Read the model definition and answer for the solid it produces. Units are mm, in the model's axes. A direction names the side the tool comes from. Coordinates: 2 decimals unless noted, no trailing zeros. Order: outer loops, then holes, each group sorted by start corner. A loop starts at its lowest first (then second) coordinate and runs counter-clockwise, first axis right, second up. Notation, with made-up numbers: (38, -38.5) - (85, -38.5) arc R28 ccw to (85, -7.5) - close; hole circle Ø7 at (-33, -30). An arc over 180 degrees is marked (long way). Write item = value, one per line.
from build123d import *

# Parameters (mm, degrees)
SKETCH_1_R      = 4.5
SKETCH_1_R_2    = 2
SKETCH_1_R_3    = 1.5
EXTRUDE_1_DEPTH = 5
SKETCH_2_R      = 15
SKETCH_2_R_2    = 1.5
SKETCH_2_R_3    = 4.5
EXTRUDE_3_DEPTH = 9.2


with BuildPart() as part:
    # 草图1 → 凸台-拉伸1 (new body)
    with BuildSketch(Plane(origin=(0, 0, 0), x_dir=(1, 0, 0), z_dir=(0, 1, 0))):
        with BuildLine():
            Line((-67.537117904, 79.170305677), (-67.537117904, -56.829694323))
            ThreePointArc((-67.537117904, -56.829694323), (-67.793701414, -58.410833153), (-68.537117904, -59.829694323))
            ThreePointArc((-68.537117904, -59.829694323), (-56.537117904, -83.829694323), (-44.537117904, -59.829694323))
            ThreePointArc((-44.537117904, -59.829694323), (-45.280534394, -58.410833153), (-45.537117904, -56.829694323))
            Line((-45.537117904, -56.829694323), (-45.537117904, 79.170305677))
            ThreePointArc((-45.537117904, 79.170305677), (-56.537117904, 90.170305677), (-67.537117904, 79.170305677))
        make_face()
        with Locations(Location((-56.537117904, 79.170305677, 0), (0, 0, 270))):
            Circle(SKETCH_1_R, mode=Mode.SUBTRACT)
        with Locations(Location((-56.537117904, 19.170305677, 0), (0, 0, 270))):
            Circle(SKETCH_1_R_2, mode=Mode.SUBTRACT)
        with Locations(Location((-56.537117904, -8.829694323, 0), (0, 0, 270))):
            Circle(SKETCH_1_R_2, mode=Mode.SUBTRACT)
        with Locations(Location((-56.537117904, -68.829694323, 0), (0, 0, 270))):
            Circle(SKETCH_1_R, mode=Mode.SUBTRACT)
        with Locations(Location((-65.197371942, -73.829694323, 0), (0, 0, 270))):
            Circle(SKETCH_1_R_3, mode=Mode.SUBTRACT)
        with Locations(Location((-47.876863866, -73.829694323, 0), (0, 0, 270))):
            Circle(SKETCH_1_R_3, mode=Mode.SUBTRACT)
        with Locations(Location((-56.537117904, -58.829694323, 0), (0, 0, 270))):
            Circle(SKETCH_1_R_3, mode=Mode.SUBTRACT)
    extrude(amount=EXTRUDE_1_DEPTH)

    # 草图2 → 凸台-拉伸3 (add)
    with BuildSketch(Plane(origin=(0, 5, 0), x_dir=(1, 0, 0), z_dir=(0, 1, 0))):
        with Locations(Location((-56.537117904, -68.829694323, 0), (0, 0, 36.869897646))):
            Circle(SKETCH_2_R)
        with Locations(Location((-65.197371942, -73.829694323, 0), (0, 0, 270))):
            Circle(SKETCH_2_R_2, mode=Mode.SUBTRACT)
        with Locations(Location((-56.537117904, -58.829694323, 0), (0, 0, 270))):
            Circle(SKETCH_2_R_2, mode=Mode.SUBTRACT)
        with Locations(Location((-47.876863866, -73.829694323, 0), (0, 0, 270))):
            Circle(SKETCH_2_R_2, mode=Mode.SUBTRACT)
        with Locations(Location((-56.537117904, -68.829694323, 0), (0, 0, 270))):
            Circle(SKETCH_2_R_3, mode=Mode.SUBTRACT)
    extrude(amount=EXTRUDE_3_DEPTH)


solid = part.part
1) The part is cut by section B-B (y = 12). Determine the outline of the cut face in (x, z).
Returned:
outline = circle Ø30 at (-56.54, 68.83); hole circle Ø3 at (-65.2, 73.83); hole circle Ø9 at (-56.54, 68.83); hole circle Ø3 at (-56.54, 58.83); hole circle Ø3 at (-47.88, 73.83)
2) The part is cut by section A-A (z = 70). Determine the outline of the cut face in (x, y), and give its area (3 significant figures).
Returned:
outline = (-71.49, 0) - (-60.88, 0) - (-60.88, 14.2) - (-71.49, 14.2) - close; (-52.19, 0) - (-41.58, 0) - (-41.58, 14.2) - (-52.19, 14.2) - close
area = 301 mm^2
3) Straight lines are drawn through the part: line 1 along Z through (x, y) = (-56.75, 6.5); line 2 along Z through (x, y) = (-55.25, 13.25); line 3 along Y through (x, z) = (-52, -28.5). For each, find the intervals that lie inside material, in ascending order. Write a range as from..to.
Returned:
line_1 = 53.83..57.34, 60.31..64.33, 73.32..83.83
line_2 = 53.89..58.06, 59.6..64.52, 73.14..83.77
line_3 = 0..5
4) The part is cut by section C-C (z = -19). Determine the outline of the cut face in (x, y), and give its area (3 significant figures).
Returned:
outline = (-67.54, 0) - (-58.53, 0) - (-58.53, 5) - (-67.54, 5) - close; (-54.54, 0) - (-45.54, 0) - (-45.54, 5) - (-54.54, 5) - close
area = 90.1 mm^2
5) The part is cut by section D-D (z = 48.5). Determine the outline of the cut face in (x, y), and give its area (3 significant figures).
Returned:
outline = (-67.54, 0) - (-45.54, 0) - (-45.54, 5) - (-67.54, 5) - close
area = 110 mm^2
6) Flat-ended cylindrical pins translate along their axes: pin 1 Ø1.5 at (x, z) = (-46, -46) entering from +Y; pin 2 Ø6 at (x, y) = (-47.5, 8.5) entering from +Z; pin 3 Ø7 at (x, z) = (-56.54, -79.17) entering from -Y; pin 4 Ø1.5 at (y, z) = (1.5, 13) entering from +X. Find the tip coordinate at first contact, or state that the pin passes through.
Returned:
pin_1 = 5
pin_2 = 82.56
pin_3 = through
pin_4 = -45.54
7) Determine the mould class of faces 1 (the face through (-56, 14.2, 64)), 2 (the face through (-67.787, 2.465, 58.389)), 3 (the face through (-66.53, 7, 74.52)), 4 (the face through (-56.339, 7.001, 64.334)) for opening direction Z: pulls with the +Z half, pulls with the -Z half, needs draft (parallel to the pull), parting line crosses it, or undercut.
Returned:
face_1 = needs draft
face_2 = pulls with the -Z half
face_3 = undercut
face_4 = undercut
8) For faces 5 (the face through (-60.584, 7.001, 83.274)), 6 (the face through (-45.537, 2, -10)), 7 (the face through (-55.185, 2.465, 7.356)), 8 (the face through (-67.537, 2, -12)), determine the directions among +Z, -Z, +X, -X, +Y, -Y from which every point of the face is accessible in a straight line to the end or side of a thin tool.
Returned:
face_5 = +Y
face_6 = -Z, +X, +Y, -Y
face_7 = +Y, -Y
face_8 = -Z, -X, +Y, -Y
